Autodesk Inventor part; units mm, degrees
ref_plane "Work Plane1" through (26.8, 0, 15.6) normal (1, 0, 0) x (0, 0, -1)
ref_plane "Work Plane2" through (28.8, 0, -15.6) normal (0, 0, -1) x (-1, 0, 0)
ref_plane "YZ Plane" through (0, 0, 0) normal (1, 0, 0) x (0, 1, 0)
sketch "Sketch2" plane through (0, 0, 0) normal (0, 1, 0) x (-1, 0, 0)
  line L0 (28.8, 15.6) -> (-28.8, 15.6)
  line L1 (-28.8, 15.6) -> (-28.8, -15.6)
  line L2 (-28.8, -15.6) -> (28.8, -15.6)
  line L3 (28.8, -15.6) -> (28.8, 15.6)
  line L4 (28.8, 15.6) -> (-28.8, -15.6) construction
  line L5 (-28.8, 15.6) -> (28.8, -15.6) construction
  circle A0 centre (7, 0) radius 1.4
  circle A1 centre (0, 0) radius 1.4
  circle A2 centre (-7, 0) radius 1.4
  dimension "d0" = 57.6
  dimension "d1" = 31.2
  dimension "d2" = 2.8
  dimension "d3" = 21.8
  dimension "d4" = 2.8
  dimension "d5" = 2.8
  dimension "d6" = 7
  dimension "d7" = 7
extrude "Extrusion1" add sketch "Sketch2" along normal blind 15
fillet "Fillet1" radius 8 2 edges at (0, 15, 15.6) (0, 15, -15.6)
ref_plane "Work Plane1" through (26.8, 0, 15.6) normal (1, 0, 0) x (0, 0, -1)
sketch "Sketch3" plane through (26.8, 0, 15.6) normal (1, 0, 0) x (0, 0, -1)
  arc A0 (8, 15) -> (0, 7) centre (8, 7) ccw
  arc A1 (8, 15) -> (0, 7) centre (8, 7) ccw
  arc A2 (8, 14) -> (1, 7) centre (8, 7) ccw
  arc A3 (31.2, 7) -> (23.2, 15) centre (23.2, 7) ccw
  arc A4 (30.2, 7) -> (23.2, 14) centre (23.2, 7) ccw
  line L0 (1, 7) -> (1, 1)
  line L1 (31.2, 0) -> (0, 0)
  line L2 (1, 1) -> (30.2, 1)
  line L3 (31.2, 0) -> (31.2, 7)
  line L4 (30.2, 1) -> (30.2, 7)
  line L5 (23.2, 15) -> (8, 15)
  line L6 (23.2, 14) -> (8, 14)
  point P0 (15.6, 0)
  dimension "d12" = 7
  dimension "d13" = 7
  dimension "d14" = 6
  dimension "d15" = 29.2
extrude "Extrusion2" cut sketch "Sketch3" against normal blind 53.6
sketch "Sketch4" plane through (0, 15, 0) normal (0, 1, 0) x (1, 0, 0)
  line L0 (26.8, -14.6) -> (26.8, 14.6)
  line L1 (-26.8, -12.5) -> (26.8, -12.5)
  line L2 (26.8, -12.5) -> (26.8, 12.5)
  line L3 (26.8, 12.5) -> (-26.8, 12.5)
  line L4 (-26.8, 12.5) -> (-26.8, -12.5)
  line L5 (-26.8, -12.5) -> (26.8, 12.5) construction
  line L6 (26.8, -12.5) -> (-26.8, 12.5) construction
  point P0 (0, 0)
  dimension "d51" = 25
extrude "Extrusion3" cut sketch "Sketch4" against normal blind 3
ref_plane "Work Plane2" through (28.8, 0, -15.6) normal (0, 0, -1) x (-1, 0, 0)
sketch "Sketch8" plane through (-26.8, 0, 15.6) normal (1, 0, 0) x (0, 0, -1)
  line L0 (3.1, 13.3238) -> (3.1, 12)
  arc A0 (3.1, 13.0156) -> (1, 7) centre (6.8512, 8.3318) ccw
  line L1 (8, 15) -> (23.2, 15)
  line L2 (15.6, 15) -> (15.6, 0.9201)
  arc A1 (30.2, 7) -> (28.1, 13.0156) centre (24.3488, 8.3318) ccw
  line L3 (28.1, 13.0156) -> (3.1, 13.0156)
  arc A2 (30.2, 7) -> (28.099, 12) centre (23.2, 7) ccw
  line L4 (1, 7) -> (30.2, 7)
  point P0 (15.6, 0)
extrude "Extrusion6" cut sketch "Sketch8" along normal blind 53.6
sketch "Sketch9" plane through (28.8, 0, -15.6) normal (0, 0, -1) x (-1, 0, 0)
  line L0 (2, 13.3238) -> (5, 13.3238)
  line L1 (5, 11.8238) -> (5, 8.2996)
  line L2 (3.5, 6.7996) -> (2, 6.7996)
  line L3 (2, 6.7996) -> (2, 13.3238)
  arc A0 (3.5, 6.7996) -> (5, 8.2996) centre (3.5, 8.2996) ccw
  arc A1 (6.5, 13.3238) -> (5, 11.8238) centre (6.5, 11.8238) ccw
  line L4 (5, 13.3238) -> (6.5, 13.3238)
  line L5 (28.8, 0) -> (28.8, 13.3238)
  line L6 (55.6, 13.3238) -> (52.6, 13.3238)
  line L7 (52.6, 11.8238) -> (52.6, 8.2996)
  line L8 (54.1, 6.7996) -> (55.6, 6.7996)
  line L9 (55.6, 6.7996) -> (55.6, 13.3238)
  arc A2 (52.6, 8.2996) -> (54.1, 6.7996) centre (54.1, 8.2996) ccw
  arc A3 (52.6, 11.8238) -> (51.1, 13.3238) centre (51.1, 11.8238) ccw
  line L10 (52.6, 13.3238) -> (51.1, 13.3238)
  line L11 (55.6, 13.3238) -> (2, 13.3238)
  line L12 (2, 7) -> (55.6, 7)
  line L13 (20.85, 13.3238) -> (36.75, 13.3238)
  line L14 (36.75, 11.8238) -> (36.75, 8.5)
  line L15 (35.25, 7) -> (22.35, 7)
  line L16 (20.85, 8.5) -> (20.85, 11.8238)
  arc A4 (20.85, 8.5) -> (22.35, 7) centre (22.35, 8.5) ccw
  arc A5 (35.25, 7) -> (36.75, 8.5) centre (35.25, 8.5) ccw
  arc A6 (38.25, 13.3238) -> (36.75, 11.8238) centre (38.25, 11.8238) ccw
  arc A7 (20.85, 11.8238) -> (19.35, 13.3238) centre (19.35, 11.8238) ccw
  line L17 (20.85, 13.3238) -> (19.35, 13.3238)
  line L18 (36.75, 13.3238) -> (38.25, 13.3238)
  point P0 (53.3509, 7)
  point P1 (4.2491, 7)
  dimension "d55" = 3
  dimension "d57" = 1.5
  dimension "d58" = 1.5
  dimension "d59" = 3
  dimension "d60" = 1.5
  dimension "d63" = 15.85
  dimension "d64" = 3
  dimension "d65" = 1.5
  dimension "d66" = 1.5
  dimension "d67" = 3
  dimension "d68" = 1.5
  dimension "d69" = 1.5
  dimension "d70" = 3
  dimension "d71" = 1.5
  dimension "d72" = 1.5
  dimension "d73" = 3
  dimension "d74" = 1.5
  dimension "d75" = 1.5
extrude "Extrusion7" cut sketch "Sketch9" against normal blind 53.8 contours L0 L4 A1 L1 A0 L12 L3 | L11 L5 L12 A4 L16 A7 | L5 L11 A6 L14 A5 L12 | A2 L7 A3 L10 L6 L9 L12
sketch "Sketch10" plane through (26.8, 1, 14.6) normal (0, 1, 0) x (1, 0, 0)
  line L0 (0, 0) -> (0, 29.2)
  line L1 (0, 14.1) -> (0, 15.1)
  line L2 (-53.6, 15.1) -> (-53.6, 14.1)
  circle A0 centre (-26.8, 14.6) radius 1.4
  line L3 (-53.6, 14.1) -> (0, 15.1) construction
  line L4 (0, 14.1) -> (-53.6, 15.1) construction
  line L5 (-37.3, 14.1) -> (-37.3, 15.1)
  circle A1 centre (-33.8, 14.6) radius 1.4
  line L6 (-16.3, 15.1) -> (-16.3, 14.1)
  circle A2 centre (-19.8, 14.6) radius 1.4
  line L7 (-53.6, 14.1) -> (-37.3, 14.1)
  line L8 (-16.3, 14.1) -> (0, 14.1)
  line L9 (0, 15.1) -> (-16.3, 15.1)
  line L10 (-37.3, 15.1) -> (-53.6, 15.1)
  dimension "d78" = 1
  dimension "d79" = 3.5
  dimension "d80" = 3.5
extrude "Extrusion8" add sketch "Sketch10" along normal blind 14 contours L8 L6 L9 L0 | L10 L5 L7 L2
sketch "Sketch11" plane through (-26.8, 1, 0.5) normal (0, 0, 1) x (1, 0, 0)
  line L0 (16.3, 14) -> (0, 14)
  line L1 (16.3, 0) -> (0, 0)
  line L2 (0, 14) -> (16.3, 0)
  line L3 (16.3, 0) -> (16.3, 14)
  line L4 (20.35, 6) -> (2.2491, 6)
  line L5 (0, 14) -> (16.3, 14)
  line L6 (16.3, 14) -> (0, 14)
  point P0 (26.8, -1)
extrude "Extrusion9" cut sketch "Sketch11" against normal blind 1
sketch "Sketch12" plane through (10.5, 1, 0.5) normal (0, 0, 1) x (1, 0, 0)
  line L0 (16.3, 0) -> (0, 0)
  line L1 (16.3, 14) -> (0, 0)
  line L2 (0, 14) -> (16.3, 14)
  line L3 (0, 0) -> (0, 14)
  line L4 (16.3, 0) -> (16.3, 14)
  line L5 (0, 14) -> (16.3, 14)
  point P0 (-10.5, -1)
extrude "Extrusion10" cut sketch "Sketch12" against normal blind 1 contours L3 L2 L1
sketch "Sketch13" plane through (28.8, 0, 15.6) normal (1, 0, 0) x (0, 0, -1)
  circle A0 centre (8, 7.8) radius 0.9
  line L0 (8, 15) -> (23.2, 15)
  line L1 (0, 0) -> (0, 7)
  line L2 (15.6, 0) -> (15.6, 15)
  line L3 (31.2, 0) -> (31.2, 7)
  circle A1 centre (23.2, 7.8) radius 0.9
  dimension "d87" = 1.8
  dimension "d88" = 7.2
  dimension "d89" = 8
  dimension "d90" = 15.6
  dimension "d91" = 15.6
extrude "Extrusion11" cut sketch "Sketch13" against normal blind 2
sketch "Sketch14" plane through (-26.8, 0, 15.6) normal (1, 0, 0) x (0, 0, -1)
  circle A0 centre (8, 7.8) radius 0.9
  circle A1 centre (8, 7.8) radius 0.9
  circle A2 centre (23.2, 7.8) radius 0.9
  circle A3 centre (23.2, 7.8) radius 0.9
  point P0 (15.6, 0)
extrude "Extrusion12" cut sketch "Sketch14" against normal blind 2
properties part number "Main body" material "ABS Plastic"
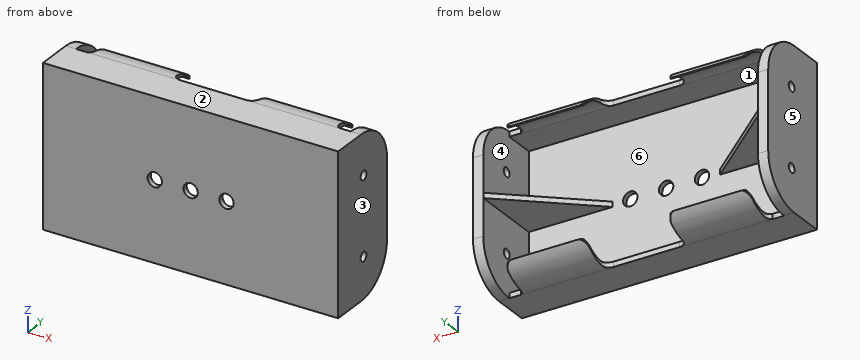
Input: part model. Units: mm. Frame: model coordinates. Face numbers are marked on the shaded views. A direction names the side the tool comes from. Give positions to 0.01 mm unless a question says otherwise; leave off trailing zeros. Order: outer loops, then holes, each group sorted by start corner. A loop starts at its lowest first (then second) coordinate and runs counter-clockwise, first axis right, second up. Notation, with made-up numbers: (42.5, 15.5) - (72.5, 15.5) arc R4 cw to (72.5, 20.5) - close; hole circle Ø3 at (51.25, 65). An arc over 180 degrees is marked (long way). Use a Markdown table: item, result.
(1) Section query D-D (x = 7). Output: boundary loops of the cut face in (y, z), then the cut area to 3 significant figures.
Computed values:
| item | result |
|---|---|
| outline | (0, -15.6) - (7, -15.6) arc R8 ccw to (7.1, -15.6) - (7.1, -14.62) arc R6 cw to (7, -14.6) - (1, -14.6) - (1, -1.4) - (0, -1.4) - close; (0, 1.4) - (1, 1.4) - (1, 14.6) - (7, 14.6) arc R6 cw to (7.1, 14.62) - (7.1, 15.6) arc R8 ccw to (7, 15.6) - (0, 15.6) - close |
| area | 40.6 mm2 |
(2) Access query for the marked faces 4, 5 and 6. Directions: +Z, -Z, +X, -X, +Y, -Y. A direction counts if a zero-diameter tool reaches every point of the face in a straight line with its end or side. Return the directions, or none.
Computed values:
| item | result |
|---|---|
| face 4 | +Y |
| face 5 | +Z, -Z, -X, +Y, -Y |
| face 6 | none |
(3) Pin query (flat end, axial travel): pin 1 (1 mm diameter, centred on x = 18, z = -3.5, fed in from +Y); pin 2 (2.5 mm diameter, centred on x = -7, z = 0, fed in from -Y); pin 3 (1.1 mm diameter, centred on x = 26, z = 15, fed in from +Y); pin 4 (2 mm diameter, centred on x = -8.5, y = 12.5, fed in from -Z). Return the tip coordinate at first contact, or that it passes through.
Computed values:
| item | result |
|---|---|
| pin 1 | stops at y = 1 |
| pin 2 | passes through |
| pin 3 | stops at y = 7 |
| pin 4 | stops at z = -14.21 |
(4) Section query C-C (y = 5.25). Output: boundary loops of the cut face in (x, z).
Computed values:
| item | result |
|---|---|
| outline | (-28.8, -15.6) - (28.8, -15.6) - (28.8, 15.6) - (-28.8, 15.6) - close; hole (-26.8, -14.6) - (26.8, -14.6) - (26.8, -0.5) - (15.45, -0.5) - (15.45, 0.5) - (26.8, 0.5) - (26.8, 14.6) - (-26.8, 14.6) - (-26.8, 0.5) - (-15.45, 0.5) - (-15.45, -0.5) - (-26.8, -0.5) - close |
(5) Section query A-A (x = 0). Output: boundary loops of the cut face in (y, z), then the cut area to 3 significant figures.
Computed values:
| item | result |
|---|---|
| outline | (0, -15.6) - (7, -15.6) - (7, -14.6) - (1, -14.6) - (1, -1.4) - (0, -1.4) - close; (0, 1.4) - (1, 1.4) - (1, 14.6) - (7, 14.6) - (7, 15.6) - (0, 15.6) - close |
| area | 40.4 mm2 |
(6) Line query: line 1 (X direction, y = 0.7, z = 0); line 2 (Z direction, x = -12.5, y = 5.5); line 3 (Z direction, x = -7, y = 0.5). Output: solid intervals per line, ascending. Write a range as from..to.
Computed values:
| item | result |
|---|---|
| line 1 | x = -28.8..-8.4, -5.6..-1.4, 1.4..5.6, 8.4..28.8 |
| line 2 | z = -15.6..-14.6, 14.6..15.6 |
| line 3 | z = -15.6..-1.4, 1.4..15.6 |
(7) Draft query along X for the marked faces 1, 2 and 3. Return one class per face: released by +X, released by -X, zero draft, split by the parting line, or undercut.
Computed values:
| item | result |
|---|---|
| face 1 | undercut |
| face 2 | zero draft |
| face 3 | released by +X |
(8) Section query B-B (z = -3). Output: boundary loops of the cut face in (x, y).
Computed values:
| item | result |
|---|---|
| outline | (-28.8, 0) - (28.8, 0) - (28.8, 15) - (26.8, 15) - (26.8, 1) - (-26.8, 1) - (-26.8, 15) - (-28.8, 15) - close |
